Can you work these out from the model? Positions are in its coordinate system, mm. Face numbers are marked on the shaded views. A direction names the side the tool comes from. Give positions to 0.01 mm unless a question says otherwise; leave off trailing zeros. Order: outer loops, then holes, each group sorted by start corner. A loop starts at its lowest first (then second) coordinate and runs counter-clockwise, first axis right, second up. Notation, with made-up numbers: (48, -16) - (86, -16) arc R22 ccw to (86, 13) - close; hole circle Ø2 at (79.25, 76). An arc over 180 degrees is marked (long way). Use one line per item in the form item = value. Start each with the question number.
1) For pin 1 (1.1 mm diameter, centred on x = -12, y = -13, fed in from -Z); pin 2 (1 mm diameter, centred on x = -1, z = 38.5, fed in from +Y), each with a flat end and sliding along its axis, tell me the tip position at first contact or that it passes through.
2) Suppose I cut it at A-A, the plane y = -13.5. Write out the boundary of the cut face in (x, z), and give its area (3 significant figures).
3) Suppose I cut it at D-D, the plane y = -4.06. Write out the boundary of the cut face in (x, z).
4) Suppose I cut it at B-B, the plane z = 8.5. Write out the boundary of the cut face in (x, y), and give its area (3 significant figures).
5) Please list where these lines run through material, in increasing order: probe 1 along X at (y, z) = (-4, 2); probe 2 along Y at (x, z) = (-10.5, 32.5); probe 3 along Z at (x, y) = (10, 13).
6) We'd pull the mould along Z, two halves only. Please class the marked faces 4, 5 and 6: released by +Z, released by -Z, zero draft, split by the parting line, or undercut.
7) Which directions (+Z, -Z, +X, -X, +Y, -Y) give clear straight access to the entire face, cutting with the end or side of a thin tool? Please do the marked faces 1, 2 and 3.
8) Suppose I cut it at C-C, the plane x = 15. Write out the boundary of the cut face in (y, z).
```python
from build123d import *

# Parameters (mm, degrees)
ESQUISSE1_W             = 40
ESQUISSE1_H             = 35.851343862
ESQUISSE1_W_2           = 32.14
ESQUISSE1_H_2           = 28.42
BOSS_EXTRU_1_DEPTH      = 39.45
ESQUISSE6_R             = 2
BOSS_EXTRU_7_DEPTH      = 7.5
ESQUISSE3_W             = 40
ESQUISSE3_H             = 35.851343862
BOSS_EXTRU_5_DEPTH      = 1.7
ENL_V_MAT_EXTRU_1_DEPTH = 0.5
ESQUISSE8_R             = 1.1
BOSS_EXTRU_8_DEPTH      = 2
CONG_1_R                = 3


with BuildPart() as part:
    # Esquisse1 → Boss.-Extru.1 (new body)
    with BuildSketch(Plane.XY):
        with Locations((0, 0.015671931)):
            Rectangle(ESQUISSE1_W, ESQUISSE1_H)
        Rectangle(ESQUISSE1_W_2, ESQUISSE1_H_2, mode=Mode.SUBTRACT)
    extrude(amount=BOSS_EXTRU_1_DEPTH)

    # Esquisse6 → Boss.-Extru.7 (add)
    with BuildSketch(Plane(origin=(0, -14.21, 0), x_dir=(1, 0, 0), z_dir=(0, 1, 0))):
        with Locations(Location((-9, -15.45, 0), (0, 0, 180))):
            Circle(ESQUISSE6_R)
        with Locations(Location((9, -15.45, 0), (0, 0, 180))):
            Circle(ESQUISSE6_R)
        with Locations(Location((-9, -29.45, 0), (0, 0, 180))):
            Circle(ESQUISSE6_R)
        with Locations(Location((9, -29.45, 0), (0, 0, 180))):
            Circle(ESQUISSE6_R)
    extrude(amount=BOSS_EXTRU_7_DEPTH)

    # Esquisse3 → Boss.-Extru.5 (add)
    with BuildSketch(Plane.XY.offset(39.45)):
        with Locations((0, 0.015671931)):
            Rectangle(ESQUISSE3_W, ESQUISSE3_H)
        Polygon((-3.144151844, -5.76), (3.144151844, -5.76), (4.277485177, -2.36), (-4.277485177, -2.36), align=None, mode=Mode.SUBTRACT)
    extrude(amount=-BOSS_EXTRU_5_DEPTH)

    # Esquisse4 → Enlèv. mat.-Extru.1 (cut)
    with BuildSketch(Plane.XY.offset(39.45)):
        with BuildLine():
            Line((-3.710818511, 0.64), (3.710818511, 0.64))
            ThreePointArc((3.710818511, 0.64), (8.410818511, -4.06), (3.710818511, -8.76))
            Line((3.710818511, -8.76), (-3.710818511, -8.76))
            ThreePointArc((-3.710818511, -8.76), (-8.410818511, -4.06), (-3.710818511, 0.64))
        make_face()
    extrude(amount=-ENL_V_MAT_EXTRU_1_DEPTH, mode=Mode.SUBTRACT)

    # Esquisse8 → Boss.-Extru.8 (add)
    # profile 1 of 2: a face of its own
    with BuildSketch(Plane(origin=(0, 0, 1.2), x_dir=(-1, 0, 0), z_dir=(0, 0, -1))):
        with BuildLine():
            Line((16.07, -10.378743894), (16.07, -14.21))
            Line((16.07, -14.21), (10.268662175, -14.21))
            Line((10.268662175, -14.21), (10.268662175, -11.778743894))
            ThreePointArc((10.268662175, -11.778743894), (10.678712682, -10.7887944), (11.668662175, -10.378743894))
            Line((11.668662175, -10.378743894), (16.07, -10.378743894))
        make_face()
        with Locations((11.668662175, -11.778743894)):
            Circle(ESQUISSE8_R, mode=Mode.SUBTRACT)
    # profile 2 of 2: a face of its own
    with BuildSketch(Plane(origin=(0, 0, 1.2), x_dir=(-1, 0, 0), z_dir=(0, 0, -1))):
        with BuildLine():
            Line((-16.07, 14.21), (-9.868662175, 14.21))
            Line((-9.868662175, 14.21), (-9.868662175, 11.778743894))
            ThreePointArc((-9.868662175, 11.778743894), (-10.395869969, 10.505951688), (-11.668662175, 9.978743894))
            Line((-11.668662175, 9.978743894), (-16.07, 9.978743894))
            Line((-16.07, 9.978743894), (-16.07, 14.21))
        make_face()
        with Locations((-11.668662175, 11.778743894)):
            Circle(ESQUISSE8_R, mode=Mode.SUBTRACT)
    extrude(amount=-BOSS_EXTRU_8_DEPTH)

    # Congé1
    cong_1_edges = [part.edges().sort_by_distance(p)[0] for p in [
        (0, -17.91, 39.45),
        (-20, -17.91, 19.725),
        (20, 0.015671931, 39.45),
        (20, -17.91, 19.725),
        (0, 17.941343862, 39.45),
        (20, 17.941343862, 19.725),
        (-20, 0.015671931, 39.45),
        (-20, 17.941343862, 19.725),
    ]]
    fillet(cong_1_edges, radius=CONG_1_R)


solid = part.part
```
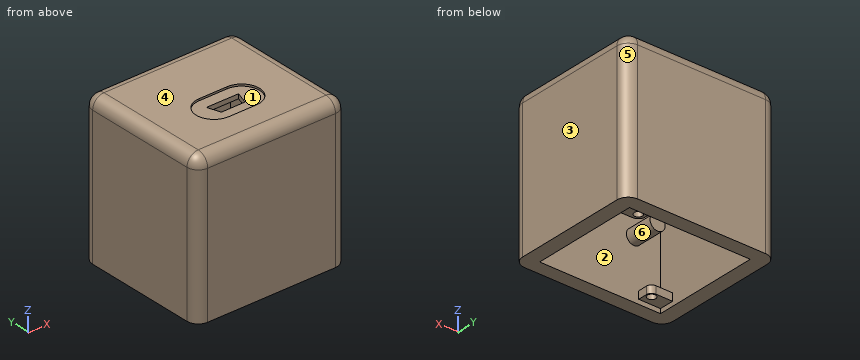
Result sheet:
q1.pin_1 = 1.2
q1.pin_2 = 17.51
q2.outline = (-20, 0) - (-16.07, 0) - (-16.07, 1.2) - (-10.27, 1.2) - (-10.27, 3.2) - (-16.07, 3.2) - (-16.07, 37.75) - (16.07, 37.75) - (16.07, 0) - (20, 0) - (20, 36.45) arc R3 ccw to (17, 39.45) - (-17, 39.45) arc R3 ccw to (-20, 36.45) - close; circle Ø4 at (-9, 15.45); circle Ø4 at (-9, 29.45); circle Ø4 at (9, 15.45); circle Ø4 at (9, 29.45)
q2.area = 423 mm²
q3.outline = (-20, 0) - (-16.07, 0) - (-16.07, 37.75) - (-3.71, 37.75) - (-3.71, 38.95) - (-8.41, 38.95) - (-8.41, 39.45) - (-17, 39.45) arc R3 ccw to (-20, 36.45) - close; (3.71, 37.75) - (16.07, 37.75) - (16.07, 0) - (20, 0) - (20, 36.45) arc R3 ccw to (17, 39.45) - (8.41, 39.45) - (8.41, 38.95) - (3.71, 38.95) - close
q4.outline = (-20, -14.91) arc R3 ccw to (-17, -17.91) - (17, -17.91) arc R3 ccw to (20, -14.91) - (20, 14.94) arc R3 ccw to (17, 17.94) - (-17, 17.94) arc R3 ccw to (-20, 14.94) - close; hole (-16.07, -14.21) - (16.07, -14.21) - (16.07, 14.21) - (-16.07, 14.21) - close
q4.area = 513 mm²
q5.probe_1 = -20 to -16.07, 16.07 to 20
q5.probe_2 = -17.91 to -14.21, 14.21 to 17.94
q5.probe_3 = 1.2 to 3.2, 37.75 to 39.45
q6.face_4 = released by +Z
q6.face_5 = zero draft
q6.face_6 = undercut
q7.face_1 = +Z
q7.face_2 = none
q7.face_3 = +Z, -Z, +X, +Y, -Y
q8.outline = (-17.91, 0) - (-14.21, 0) - (-14.21, 37.75) - (14.21, 37.75) - (14.21, 3.2) - (9.98, 3.2) - (9.98, 1.2) - (14.21, 1.2) - (14.21, 0) - (17.94, 0) - (17.94, 36.45) arc R3 ccw to (14.94, 39.45) - (-14.91, 39.45) arc R3 ccw to (-17.91, 36.45) - close
